Verification items for the finished model (mm, model axes). Round coordinates to 2 decimals unless told otherwise and drop trailing zeros. Loops run counter-clockwise (first coordinate to the right, second up) from the corner with the lowest first, then second, coordinate; pieces in that order, holes last. Notation, with made-up numbers: (65.5, 39) -> (122.5, 39) arc R31 ccw to (122.5, 69) -> close; hole circle Ø10 at (-3.75, 60). An arc over 180 degrees is marked (long way). Use CSV: the item, a comma, the result in double quotes. Start each with the question number.
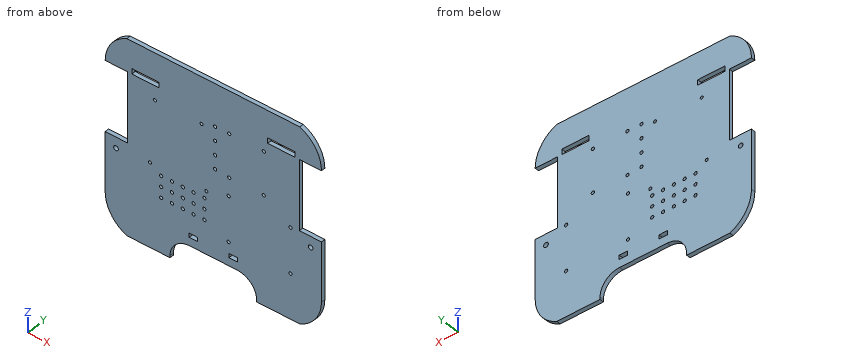
```python
from build123d import *

# Parameters (mm, degrees)
SKETCH1_W           = 254
SKETCH1_H           = 228.6
BOSS_EXTRUDE1_DEPTH = 4.826
SKETCH2_W           = 26.00000007
SKETCH2_H           = 82.55
CUT_EXTRUDE1_DEPTH  = 4.826
CUT_EXTRUDE3_DEPTH  = 4.826
SKETCH7_W           = 50.8
SKETCH7_H           = 25.4
CUT_EXTRUDE5_DEPTH  = 4.826
FILLET9_R           = 22.86
FILLET10_R          = 22.86
CUT_EXTRUDE6_DEPTH  = 4.826
SKETCH9_W           = 31.75
SKETCH9_H           = 6.35
CUT_EXTRUDE7_DEPTH  = 171.929167423
SKETCH11_W          = 9.906
SKETCH11_H          = 4.826
CUT_EXTRUDE8_DEPTH  = 171.929167423
SKETCH13_R          = 1.905
CUT_EXTRUDE10_DEPTH = 171.929167423
SKETCH14_R          = 1.778
CUT_EXTRUDE11_DEPTH = 171.929167423
SKETCH15_R          = 1.905
CUT_EXTRUDE12_DEPTH = 171.929167423
SKETCH16_R          = 1.905
CUT_EXTRUDE13_DEPTH = 171.929167423
SKETCH17_R          = 2.778125
CUT_EXTRUDE14_DEPTH = 171.929167423
SKETCH18_R          = 1.905
CUT_EXTRUDE15_DEPTH = 171.929167423


with BuildPart() as part:
    # Sketch1 → Boss-Extrude1 (new body)
    with BuildSketch(Plane(origin=(0, 0, 0), x_dir=(1, 0, 0), z_dir=(0, 1, 0))):
        Rectangle(SKETCH1_W, SKETCH1_H)
    extrude(amount=BOSS_EXTRUDE1_DEPTH)

    # Sketch2 → Cut-Extrude1 (cut)
    with BuildSketch(Plane(origin=(0, 4.826, 0), x_dir=(1, 0, 0), z_dir=(0, 1, 0))):
        with Locations((-113.999999965, -34.925)):
            Rectangle(SKETCH2_W, SKETCH2_H)
        with Locations((113.999999965, -34.925)):
            Rectangle(SKETCH2_W, SKETCH2_H)
    extrude(amount=-CUT_EXTRUDE1_DEPTH, mode=Mode.SUBTRACT)

    # Sketch4 → Cut-Extrude3 (cut)
    with BuildSketch(Plane(origin=(0, 4.826, 0), x_dir=(1, 0, 0), z_dir=(0, 1, 0))):
        with BuildLine():
            Line((-127, 76.2), (-127, 114.3))
            Line((-127, 114.3), (-101.6, 114.3))
            ThreePointArc((-101.6, 114.3), (-120.067875899, 99.095250599), (-127, 76.2))
        make_face()
        with BuildLine():
            Line((127, 76.2), (127, 114.3))
            Line((127, 114.3), (101.6, 114.3))
            ThreePointArc((101.6, 114.3), (120.067875899, 99.095250599), (127, 76.2))
        make_face()
    extrude(amount=-CUT_EXTRUDE3_DEPTH, mode=Mode.SUBTRACT)

    # Sketch7 → Cut-Extrude5 (cut)
    with BuildSketch(Plane(origin=(0, 4.826, 0), x_dir=(1, 0, 0), z_dir=(0, 1, 0))):
        with Locations((-25.4, 101.6)):
            Rectangle(SKETCH7_W, SKETCH7_H)
        with Locations((25.4, 101.6)):
            Rectangle(SKETCH7_W, SKETCH7_H)
    extrude(amount=-CUT_EXTRUDE5_DEPTH, mode=Mode.SUBTRACT)

    # Fillet9
    fillet9_edges = [part.edges().sort_by_distance(p)[0] for p in [
        (-50.8, 2.413, -88.9),
    ]]
    fillet(fillet9_edges, radius=FILLET9_R)

    # Fillet10
    fillet10_edges = [part.edges().sort_by_distance(p)[0] for p in [
        (50.8, 2.413, -88.9),
    ]]
    fillet(fillet10_edges, radius=FILLET10_R)

    # Sketch8 → Cut-Extrude6 (cut)
    with BuildSketch(Plane(origin=(0, 4.826, 0), x_dir=(1, 0, 0), z_dir=(0, 1, 0))):
        with BuildLine():
            Line((-127, -76.2), (-127, -114.3))
            Line((-127, -114.3), (-101.6, -114.3))
            ThreePointArc((-101.6, -114.3), (-120.067875899, -99.095250599), (-127, -76.2))
        make_face()
        with BuildLine():
            Line((127, -114.3), (101.6, -114.3))
            ThreePointArc((101.6, -114.3), (120.067875899, -99.095250599), (127, -76.2))
            Line((127, -76.2), (127, -114.3))
        make_face()
    extrude(amount=-CUT_EXTRUDE6_DEPTH, mode=Mode.SUBTRACT)

    # Sketch9 → Cut-Extrude7 (cut, through all)
    with BuildSketch(Plane.XZ):
        with Locations((-79.79099993, 79.375)):
            Rectangle(SKETCH9_W, SKETCH9_H)
        with Locations((79.79099993, 79.375)):
            Rectangle(SKETCH9_W, SKETCH9_H)
    extrude(amount=-CUT_EXTRUDE7_DEPTH, mode=Mode.SUBTRACT)

    # Sketch11 → Cut-Extrude8 (cut, through all)
    with BuildSketch(Plane(origin=(0, 4.826, 0), x_dir=(1, 0, 0), z_dir=(0, 1, 0))):
        with Locations((-23.345869789, 76.863822677)):
            Rectangle(SKETCH11_W, SKETCH11_H)
        with Locations((23.345869789, 76.863822677)):
            Rectangle(SKETCH11_W, SKETCH11_H)
    extrude(amount=-CUT_EXTRUDE8_DEPTH, mode=Mode.SUBTRACT)

    # Sketch13 → Cut-Extrude10 (cut, through all)
    with BuildSketch(Plane(origin=(0, 4.826, 0), x_dir=(1, 0, 0), z_dir=(0, 1, 0))):
        with Locations(Location((-10.4749371, 24.715879034, 0), (0, 0, 270))):
            Circle(SKETCH13_R)
        with Locations(Location((-23.1749371, 24.715879034, 0), (0, 0, 270))):
            Circle(SKETCH13_R)
        with Locations(Location((-35.8749371, 24.715879034, 0), (0, 0, 270))):
            Circle(SKETCH13_R)
        with Locations(Location((-48.5749371, 24.715879034, 0), (0, 0, 270))):
            Circle(SKETCH13_R)
        with Locations(Location((-61.2749371, 24.715879034, 0), (0, 0, 270))):
            Circle(SKETCH13_R)
        with Locations(Location((-23.1749371, 37.415879034, 0), (0, 0, 270))):
            Circle(SKETCH13_R)
        with Locations(Location((-35.8749371, 37.415879034, 0), (0, 0, 270))):
            Circle(SKETCH13_R)
        with Locations(Location((-48.5749371, 37.415879034, 0), (0, 0, 270))):
            Circle(SKETCH13_R)
        with Locations(Location((-61.2749371, 37.415879034, 0), (0, 0, 270))):
            Circle(SKETCH13_R)
        with Locations(Location((-23.1749371, 50.115879034, 0), (0, 0, 270))):
            Circle(SKETCH13_R)
        with Locations(Location((-35.8749371, 50.115879034, 0), (0, 0, 270))):
            Circle(SKETCH13_R)
        with Locations(Location((-48.5749371, 50.115879034, 0), (0, 0, 270))):
            Circle(SKETCH13_R)
        with Locations(Location((-61.2749371, 50.115879034, 0), (0, 0, 270))):
            Circle(SKETCH13_R)
        with Locations(Location((-10.4749371, 37.415879034, 0), (0, 0, 270))):
            Circle(SKETCH13_R)
        with Locations(Location((-10.4749371, 50.115879034, 0), (0, 0, 270))):
            Circle(SKETCH13_R)
    extrude(amount=-CUT_EXTRUDE10_DEPTH, mode=Mode.SUBTRACT)

    # Sketch14 → Cut-Extrude11 (cut, through all)
    with BuildSketch(Plane(origin=(0, 4.826, 0), x_dir=(1, 0, 0), z_dir=(0, 1, 0))):
        with Locations(Location((-68.6409371, -59.556843517, 0), (0, 0, 270))):
            Circle(SKETCH14_R)
        with Locations(Location((-13.7769371, -59.556843517, 0), (0, 0, 270))):
            Circle(SKETCH14_R)
        with Locations(Location((-74.4829371, 15.627156483, 0), (0, 0, 270))):
            Circle(SKETCH14_R)
        with Locations(Location((-8.1889371, 15.627156483, 0), (0, 0, 270))):
            Circle(SKETCH14_R)
    extrude(amount=-CUT_EXTRUDE11_DEPTH, mode=Mode.SUBTRACT)

    # Sketch15 → Cut-Extrude12 (cut, through all)
    with BuildSketch(Plane(origin=(0, 4.826, 0), x_dir=(1, 0, 0), z_dir=(0, 1, 0))):
        with Locations(Location((59.276921846, -64.485146072, 0), (0, 0, 270))):
            Circle(SKETCH15_R)
        with Locations(Location((18.636921846, -64.485146072, 0), (0, 0, 270))):
            Circle(SKETCH15_R)
        with Locations(Location((59.276921846, -13.685146072, 0), (0, 0, 270))):
            Circle(SKETCH15_R)
        with Locations(Location((18.636921846, -13.685146072, 0), (0, 0, 270))):
            Circle(SKETCH15_R)
    extrude(amount=-CUT_EXTRUDE12_DEPTH, mode=Mode.SUBTRACT)

    # Sketch16 → Cut-Extrude13 (cut, through all)
    with BuildSketch(Plane(origin=(0, 4.826, 0), x_dir=(1, 0, 0), z_dir=(0, 1, 0))):
        with Locations(Location((90.645921846, 7.99943228, 0), (0, 0, 270))):
            Circle(SKETCH16_R)
        with Locations(Location((18.001921846, 7.99943228, 0), (0, 0, 270))):
            Circle(SKETCH16_R)
        with Locations(Location((18.001921846, 61.33943228, 0), (0, 0, 270))):
            Circle(SKETCH16_R)
        with Locations(Location((90.645921846, 61.33943228, 0), (0, 0, 270))):
            Circle(SKETCH16_R)
    extrude(amount=-CUT_EXTRUDE13_DEPTH, mode=Mode.SUBTRACT)

    # Sketch17 → Cut-Extrude14 (cut, through all)
    with BuildSketch(Plane.XZ):
        with Locations(Location((114.3, -19.164632523, 0), (0, 0, 270))):
            Circle(SKETCH17_R)
        with Locations(Location((-114.3, -19.164632523, 0), (0, 0, 270))):
            Circle(SKETCH17_R)
    extrude(amount=-CUT_EXTRUDE14_DEPTH, mode=Mode.SUBTRACT)

    # Sketch18 → Cut-Extrude15 (cut, through all)
    with BuildSketch(Plane(origin=(0, 4.826, 0), x_dir=(1, 0, 0), z_dir=(0, 1, 0))):
        with Locations(Location((2.126921846, -64.485146072, 0), (0, 0, 270))):
            Circle(SKETCH18_R)
        with Locations(Location((2.126921846, -47.975146072, 0), (0, 0, 270))):
            Circle(SKETCH18_R)
        with Locations(Location((2.126921846, -31.465146072, 0), (0, 0, 270))):
            Circle(SKETCH18_R)
        with Locations(Location((2.126921846, -14.955146072, 0), (0, 0, 270))):
            Circle(SKETCH18_R)
    extrude(amount=-CUT_EXTRUDE15_DEPTH, mode=Mode.SUBTRACT)


solid = part.part
```
Q1. Thickness scan on L1, parallel to Z at x = 58, y = 0.2; L2, parallel to X at y = 4.6, z = 77.5; L3, parallel to Z at x = -94, y = 0.3. Record the ranges inside material, lowest first. Write a range as from..to.
Q2. Cross-section at C-C (y = 3.9). State how many separate pieces and enclosed holes the cut face has, and give its area (3 significant figures).
Q3. Cross-section at A-A (x = -91.5). Record the boundary of the cut face in (y, z), and give its area (3 significant figures).
Q4. Cross-section at B-B (x = 114.3). Record the boundary of the cut face in (y, z).
Q5. Depth check by flat-ended pin: pin 1 Ø1.4 at (y, z) = (2.5, -77.5) entering from -X. Enter the tip coordinate at first touch or a pass-through.
Q6. Cross-section at D-D (x = 8). Record the boundary of the cut face in (y, z), and give its area (3 significant figures).
Answer list:
1,L1,"z = -114.3..12.27, 15.1..63.07, 65.9..114.3"
1,L2,"x = -126.98..-95.67, -63.92..63.92, 95.67..126.98"
1,L3,"z = -114.3..76.2, 82.55..114.3"
2,separate pieces,"1"
2,enclosed holes,"37"
2,area,"49,400 mm2"
3,outline,"(0, -114.3) -> (4.83, -114.3) -> (4.83, 76.2) -> (0, 76.2) -> close; (0, 82.55) -> (4.83, 82.55) -> (4.83, 114.3) -> (0, 114.3) -> close"
3,area,"1,070 mm2"
4,outline,"(0, -105.98) -> (4.83, -105.98) -> (4.83, -21.94) -> (0, -21.94) -> close; (0, -16.39) -> (4.83, -16.39) -> (4.83, -6.35) -> (0, -6.35) -> close; (0, 76.2) -> (4.83, 76.2) -> (4.83, 105.98) -> (0, 105.98) -> close"
5,pin 1,"stops at x = -127"
6,outline,"(0, -88.9) -> (4.83, -88.9) -> (4.83, 114.3) -> (0, 114.3) -> close"
6,area,"981 mm2"
